Verification items for the finished model (mm, model axes). Coordinates: 2 decimals unless noted, no trailing zeros. Write each loop counter-clockwise with the first axis right and the second up, starting at its lowest first coordinate (ties: lowest second). Pieces come first, ordered by that corner, then holes. Notation, with made-up numbers: (75.25, 74) -> (123.25, 74) arc R31 ccw to (123.25, 111) -> close; hole circle Ø6 at (50.5, 15.25). An arc over 180 degrees is marked (long way). Answer in a Markdown table with one row per item.
```python
from build123d import *
from OCP.BRepFilletAPI import BRepFilletAPI_MakeChamfer

# Parameters (mm, degrees)
SKETCH1_R           = 36.5
SKETCH1_R_2         = 25
BOSS_EXTRUDE1_DEPTH = 130
CHAMFER1_SIZE       = 3
CHAMFER1_SIZE2      = 5.196152423
CHAMFER2_SIZE       = 2
CHAMFER2_SIZE2      = 7.464101615
CHAMFER3_SIZE       = 2
CHAMFER3_SIZE2      = 7.464101615


with BuildPart() as part:
    # Sketch1 → Boss-Extrude1 (new body)
    with BuildSketch(Plane(origin=(0, 0, 0), x_dir=(1, 0, 0), z_dir=(0, 1, 0))):
        with Locations(Location((0, 0, 0), (0, 0, 270))):
            Circle(SKETCH1_R)
        with Locations(Location((0, 0, 0), (0, 0, 270))):
            Circle(SKETCH1_R_2, mode=Mode.SUBTRACT)
    extrude(amount=-BOSS_EXTRUDE1_DEPTH)

    # Chamfer1: one chamfer whose edges measure the first distance from different faces: ONE call of the kernel's chamfer builder (chamfer() names one face for all edges)
    chamfer1_edges_1 = [part.edges().sort_by_distance(p)[0] for p in [
        (0, -130, -25),
    ]]
    chamfer1_side_1 = [part.faces().sort_by_distance(p)[0] for p in [
        (0, -65, -25),
    ]]
    chamfer1_edges_2 = [part.edges().sort_by_distance(p)[0] for p in [
        (0, 0, -25),
    ]]
    chamfer1_side_2 = [part.faces().sort_by_distance(p)[0] for p in [
        (0, 0, -35.467624099),
    ]]
    chamfer1 = BRepFilletAPI_MakeChamfer(part.part.solid().wrapped)
    for e in chamfer1_edges_1:
        chamfer1.Add(CHAMFER1_SIZE, CHAMFER1_SIZE2, e.wrapped, chamfer1_side_1[0].wrapped)  # the first distance lies on this face
    for e in chamfer1_edges_2:
        chamfer1.Add(CHAMFER1_SIZE, CHAMFER1_SIZE2, e.wrapped, chamfer1_side_2[0].wrapped)  # the first distance lies on this face
    add(Compound.cast(chamfer1.Shape()), mode=Mode.REPLACE)

    # Chamfer2
    chamfer2_edges = [part.edges().sort_by_distance(p)[0] for p in [
        (0, -130, -36.5),
    ]]
    chamfer2_side = [part.faces().sort_by_distance(p)[0] for p in [
        (0, -130, -31.228528323),
    ]]
    chamfer(chamfer2_edges, length=CHAMFER2_SIZE, length2=CHAMFER2_SIZE2, reference=chamfer2_side[0])

    # Chamfer3
    chamfer3_edges = [part.edges().sort_by_distance(p)[0] for p in [
        (0, 0, -36.5),
    ]]
    chamfer3_side = [part.faces().sort_by_distance(p)[0] for p in [
        (0, 0, -29.032375901),
    ]]
    chamfer(chamfer3_edges, length=CHAMFER3_SIZE, length2=CHAMFER3_SIZE2, reference=chamfer3_side[0])


solid = part.part
```
1. Sectioned sample at B-B, the plane x = 0. Record the cut outline in (y, z), and give its area (3 significant figures).
Findings below:
| item | result |
|---|---|
| outline | (-130, -34.5) -> (-122.54, -36.5) -> (-7.46, -36.5) -> (0, -34.5) -> (0, -28) -> (-5.2, -25) -> (-127, -25) -> (-130, -30.2) -> close; (-130, 30.2) -> (-127, 25) -> (-5.2, 25) -> (0, 28) -> (0, 34.5) -> (-7.46, 36.5) -> (-122.54, 36.5) -> (-130, 34.5) -> close |
| area | 2,930 mm² |
2. Go/stop test with flat-tipped pins: pin 1 (6 mm diameter, centred on x = -11, y = -72.5, fed in from +Z); pin 2 (10 mm diameter, centred on y = -50, z = 14.5, fed in from +X); pin 3 (6 mm diameter, centred on y = -80.5, z = -2.5, fed in from +X). Record where each tip stops, or that it passes through.
Findings below:
| item | result |
|---|---|
| pin 1 | stops at z = 35.61 |
| pin 2 | stops at x = 35.24 |
| pin 3 | stops at x = 36.5 |
3. Sectioned sample at C-C, the plane y = -10. Record the cut outline in (x, z), and give its area (3 significant figures).
Findings below:
| item | result |
|---|---|
| outline | circle Ø73 at (0, 0); hole circle Ø50 at (0, 0) |
| area | 2,220 mm² |
4. Material ranges on probe 1 along X at (y, z) = (-75.5, 0); probe 2 along Z at (x, y) = (-20, -91.5); probe 3 along Z at (x, y) = (14, -76), recorded low to high. Write a range as from..to.
Findings below:
| item | result |
|---|---|
| probe 1 | x = -36.5..-25, 25..36.5 |
| probe 2 | z = -30.53..-15, 15..30.53 |
| probe 3 | z = -33.71..-20.71, 20.71..33.71 |
5. Sectioned sample at A-A, the plane z = 0. Record the cut outline in (x, y), and give its area (3 significant figures).
Findings below:
| item | result |
|---|---|
| outline | (-36.5, -122.54) -> (-34.5, -130) -> (-30.2, -130) -> (-25, -127) -> (-25, -5.2) -> (-28, 0) -> (-34.5, 0) -> (-36.5, -7.46) -> close; (25, -127) -> (30.2, -130) -> (34.5, -130) -> (36.5, -122.54) -> (36.5, -7.46) -> (34.5, 0) -> (28, 0) -> (25, -5.2) -> close |
| area | 2,930 mm² |
6. Release check for a two-part mould opening along X. For faces 1 (the face through (28.3, 0, -0.2)), 2 (the face through (-33.8, -129.53, -7.51)), 3 (the face through (-24.55, -4.94, -5.45)), 4 (the face through (7.509, -65.245, 23.846)) record: released by +X, released by -X, zero draft, split by the parting line, or undercut.
Findings below:
| item | result |
|---|---|
| face 1 | zero draft |
| face 2 | split by the parting line |
| face 3 | undercut |
| face 4 | undercut |
